Work out the finished part from the listing and answer in its coordinate system (mm). Face numbers are marked on the shaded views. A direction names the side the tool comes from. Round coordinates to 2 decimals unless told otherwise and drop trailing zeros. Loops run counter-clockwise (first coordinate to the right, second up) from the corner with the lowest first, then second, coordinate; pieces in that order, holes last. Notation, with made-up numbers: M -9,30.5 L 6,30.5 A12 ccw 6,45.5 Z; hole C 44.25,28 d4. An arc over 180 degrees is marked long. One line per item, written item: value.
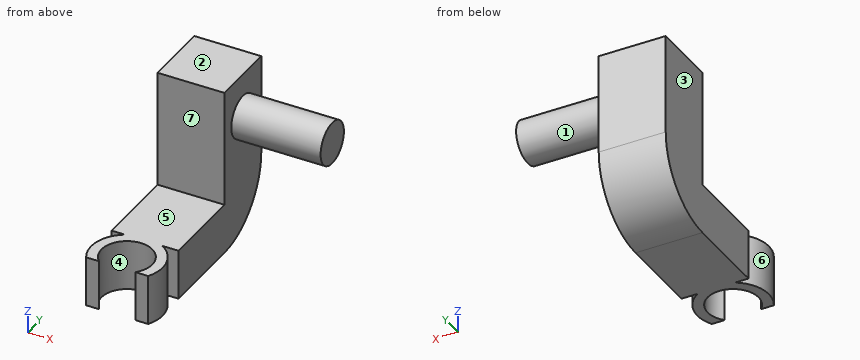
```python
from build123d import *

# Parameters (mm, degrees)
F0_W      = 5.08
F0_H      = 12.7
F1_DEPTH  = 5.08
F2_W      = 5.08
F2_H      = 3.81
F3_DEPTH  = 6.35
F4_R      = 5.08
F5_R      = 2.7121475218
F6_DEPTH  = 3.81
F7_R      = 1.9253373718
F8_DEPTH  = 3.81
F9_W      = 5.3527112813
F9_H      = 1.6279429131
F10_DEPTH = 3.81
F11_SCALE = 1.5
F12_R     = 2.413
F13_DEPTH = 10.16


with BuildPart() as f1:
    # F0 (on Front) → F1 (new body)
    with BuildSketch(Plane.XZ):
        with Locations((2.54, 20.2292869008)):
            Rectangle(F0_W, F0_H)
    extrude(amount=F1_DEPTH)

    # F2 (on face) → F3 (join)
    with BuildSketch(Plane.XZ.offset(5.08)):
        with Locations((2.54, 15.7842869008)):
            Rectangle(F2_W, F2_H)
    extrude(amount=F3_DEPTH)

    # F4
    f4_edges = [f1.edges().sort_by_distance(p)[0] for p in [
        (2.54, 0, 13.879287),
    ]]
    fillet(f4_edges, radius=F4_R)

    # F5 (on face) → F6 (join)
    with BuildSketch(Plane.XY.offset(17.6892869008)):
        with Locations((2.4383503072, -13.7368525874)):
            Circle(F5_R)
    extrude(amount=-F6_DEPTH)

    # F7 (on face) → F8 (cut)
    with BuildSketch(Plane.XY.offset(17.6892869008)):
        with Locations((2.4383503072, -13.7368525874)):
            Circle(F7_R)
    extrude(amount=-F8_DEPTH, mode=Mode.SUBTRACT)

    # F9 (on face) → F10 (cut)
    with BuildSketch(Plane.XY.offset(17.6892869008)):
        with Locations((2.7606785416, -15.8977832678)):
            Rectangle(F9_W, F9_H)
    extrude(amount=-F10_DEPTH, mode=Mode.SUBTRACT)


with BuildPart() as f1_1:
    # F11: moved
    add(f1.part.scale(F11_SCALE))

    # F12 (on face) → F13 (join)
    with BuildSketch(Plane.YZ.offset(7.62)):
        with Locations((-3.81, 34.9159303513)):
            Circle(F12_R)
    extrude(amount=F13_DEPTH)


solid = f1_1.part
```
1) Each of these flat-tipped pins is pushed along its axis until it touches: pin 1 (6 mm diameter, centred on x = 14, y = -4, fed in from -Z); pin 2 (2.5 mm diameter, centred on x = 4.5, z = 32.5, fed in from -Y); pin 3 (5 mm diameter, centred on y = -10, z = 26, fed in from +X); pin 4 (1 mm diameter, centred on x = 15, z = 30.5, fed in from -Y). Where does it stop, or does it pass through?
Check values:
pin 1: z = 32.5
pin 2: y = -7.62
pin 3: x = 7.62
pin 4: through
2) Find section C-C (x = 2.5). Give the vertices of the cut face in (y, z).
Check values:
outline: M -17.96,20.82 L -7.62,20.82 A7.62 ccw 0,28.44 L 0,39.87 L -7.62,39.87 L -7.62,26.53 L -17.96,26.53 Z
3) Find the intervals of material crossed by probe 1 along X at (y, z) = (-18, 24.5); probe 2 along X at (y, z) = (-13.75, 24.75); probe 3 along Y at (x, z) = (4.5, 38), in increasing order. Write a range as from..to.
Check values:
probe 1: 0.53..2.41, 4.9..6.78
probe 2: 0..7.62
probe 3: -7.62..0
4) Find section B-B (z = 37). Give the vertices of the cut face in (x, y).
Check values:
outline: M 0,-7.62 L 7.62,-7.62 L 7.62,-5.03 L 17.78,-5.03 L 17.78,-2.59 L 7.62,-2.59 L 7.62,0 L 0,0 Z
5) For the marked faces 1, 2 and 3, determine the directions among +Z, -Z, +X, -X, +Y, -Y from which every point of the face is accessible in a straight line to the end or side of a thin tool.
Check values:
face 1: +X
face 2: +Z, +X, -X, +Y, -Y
face 3: +Z, -Z, -X, +Y
6) The mould has two halves that part along Y. Classify the marked faces 4, 5, 6 and 7: +Y half, -Y half, draft (parallel to the pull), parting line (faces both ways), or undercut.
Check values:
face 4: undercut
face 5: draft
face 6: undercut
face 7: -Y half
7) Find section A-A (y = -18). Give the vertices of the cut face in (x, z).
Check values:
outline: M 0.53,20.82 L 2.41,20.82 L 2.41,26.53 L 0.53,26.53 Z; M 4.9,20.82 L 6.78,20.82 L 6.78,26.53 L 4.9,26.53 Z
8) Find section D-D (y = -3.81). Give the vertices of the cut face in (x, z).
Check values:
outline: M 0,21.84 L 7.62,21.84 L 7.62,32.5 L 17.78,32.5 L 17.78,37.33 L 7.62,37.33 L 7.62,39.87 L 0,39.87 Z
